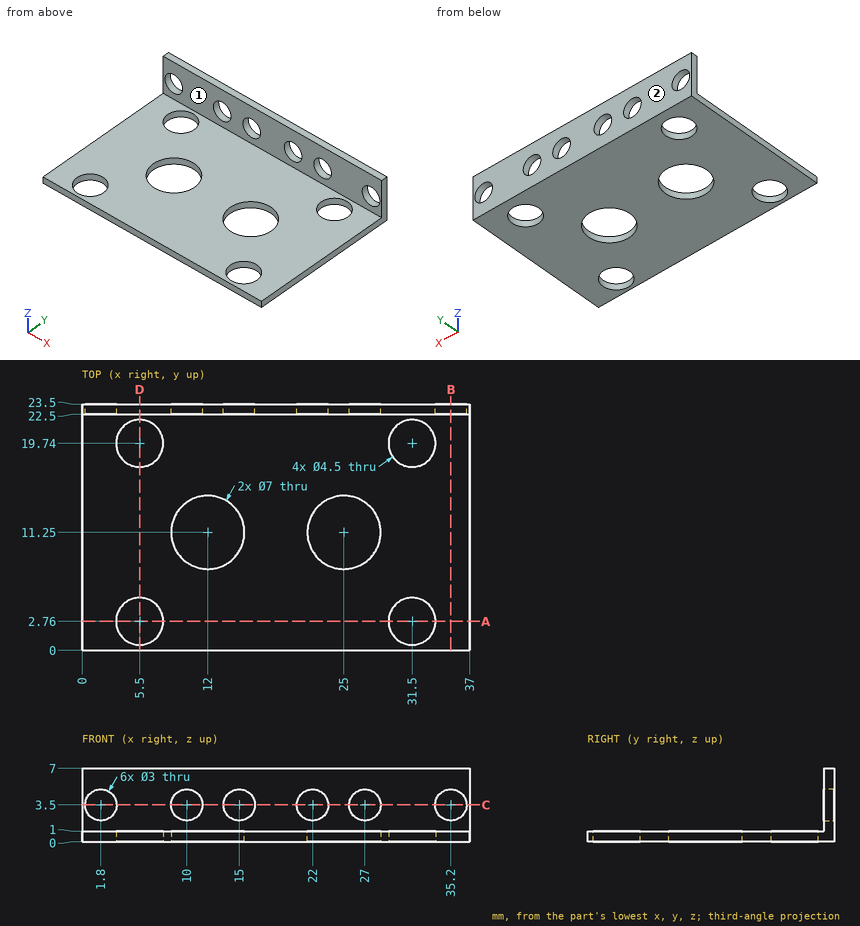
Source: three-view drawing plus pictorial views. Frame: mm from the lowest corner of the part. A direction names the side the tool comes from. Round coordinates to 2 decimals unless told otherwise and drop trailing zeros. Loops run counter-clockwise (first coordinate to the right, second up) from the corner with the lowest first, then second, coordinate; pieces in that order, holes last.
Item 1: Reachability of the marked faces 1 and 2 from +Z, -Z, +X, -X, +Y, -Y: full face, straight path, thin tool, end or side. Return the list, or none.
Checked values:
face 1: +Z, +X, -X, -Y
face 2: +Z, -Z, +X, -X, +Y
Item 2: Section D-D, the plane x = 5.5. Output: boundary loops of the cut face in (y, z).
Checked values:
outline: (0, 0) - (0.51, 0) - (0.51, 1) - (0, 1) - close; (5.01, 0) - (17.49, 0) - (17.49, 1) - (5.01, 1) - close; (21.99, 0) - (23.5, 0) - (23.5, 7) - (22.5, 7) - (22.5, 1) - (21.99, 1) - close
Item 3: Section A-A, the plane y = 2.76. Output: boundary loops of the cut face in (x, z).
Checked values:
outline: (0, 0) - (3.25, 0) - (3.25, 1) - (0, 1) - close; (7.75, 0) - (29.25, 0) - (29.25, 1) - (7.75, 1) - close; (33.75, 0) - (37, 0) - (37, 1) - (33.75, 1) - close
Item 4: Section C-C, the plane z = 3.5. Output: boundary loops of the cut face in (x, y).
Checked values:
outline: (0, 22.5) - (0.3, 22.5) - (0.3, 23.5) - (0, 23.5) - close; (3.3, 22.5) - (8.5, 22.5) - (8.5, 23.5) - (3.3, 23.5) - close; (11.5, 22.5) - (13.5, 22.5) - (13.5, 23.5) - (11.5, 23.5) - close; (16.5, 22.5) - (20.5, 22.5) - (20.5, 23.5) - (16.5, 23.5) - close; (23.5, 22.5) - (25.5, 22.5) - (25.5, 23.5) - (23.5, 23.5) - close; (28.5, 22.5) - (33.7, 22.5) - (33.7, 23.5) - (28.5, 23.5) - close; (36.7, 22.5) - (37, 22.5) - (37, 23.5) - (36.7, 23.5) - close
Item 5: Section B-B, the plane x = 35.2. Output: boundary loops of the cut face in (y, z), plus the area to 3 significant figures.
Checked values:
outline: (0, 0) - (23.5, 0) - (23.5, 2) - (22.5, 2) - (22.5, 1) - (0, 1) - close; (22.5, 5) - (23.5, 5) - (23.5, 7) - (22.5, 7) - close
area: 26.5 mm2
Item 6: Contact query for flat-ended pins moving along their axis: P1, Ø1, axis at x = 22.5, z = 2.5, coming from the -Y side; P2, Ø8, axis at x = 8, y = 15, coming from the +Z side; P3, Ø7, axis at x = 31.5, y = 19.74, coming from the -Z side. Output: stop coordinate, or through.
Checked values:
P1: stops at y = 22.5
P2: stops at z = 1
P3: stops at z = 0
Item 7: Line query: L1, parallel to Y at x = 5.5, z = 0.5; L2, parallel to Y at x = 12, z = 0.5; L3, parallel to Y at x = 16.5, z = 5.75. Output: solid intervals per line, ascending.
Checked values:
L1: y = 0 to 0.51, 5.01 to 17.49, 21.99 to 23.5
L2: y = 0 to 7.75, 14.75 to 23.5
L3: y = 22.5 to 23.5
